Can you work these out from the model? Positions are in its coordinate system, mm. Face numbers are marked on the shaded views. A direction names the side the tool comes from. Give positions to 0.01 mm unless a question says otherwise; leave off trailing zeros. Write each loop counter-clockwise with the first axis right and the second up, starting at its lowest first coordinate (ties: lowest second). Pieces come first, ordered by that corner, then holes.
1. Suppose I cut it at A-A (z = 14.5). Please give me the cut outline in (x, y), and give its area (3 significant figures).
2. On a 3-axis mill with a long thin cutter (end or side, diameter ignored), from which of +Z, -Z, +X, -X, +Y, -Y can I reach the whole of each face in a straight line? I mean the marked faces 4, 5 and 6. Say none if no direction works.
3. I'm going to push flat-ended pins straight in: pin 1 (17.5 mm diameter, centred on x = 121.5, y = 19, fed in from +Z); pin 2 (6 mm diameter, centred on x = 19.5, y = 13.5, fed in from -Z); pin 3 (20.5 mm diameter, centred on x = 63.5, z = 59.69, fed in from -Y); pin 4 (8 mm diameter, centred on y = 51.5, z = 42.5, fed in from -X). Where does each tip first touch, or does it pass through?
4. Thinking about a two-plate mould opening in Z: for the marked faces 1, 2 and 3, which applies, pulls with the +Z half, pulls with the -Z half, needs draft (parallel to the pull), parting line crosses it, or undercut?
5. If I drill on probe 1 along Y at (x, z) = (63.5, 76.5) (3 decimals); probe 2 along X at (y, z) = (38, 9.5); probe 3 along Z at (x, y) = (21.5, 47.5), over which ranges is the centre line in solid material (lowest first)?
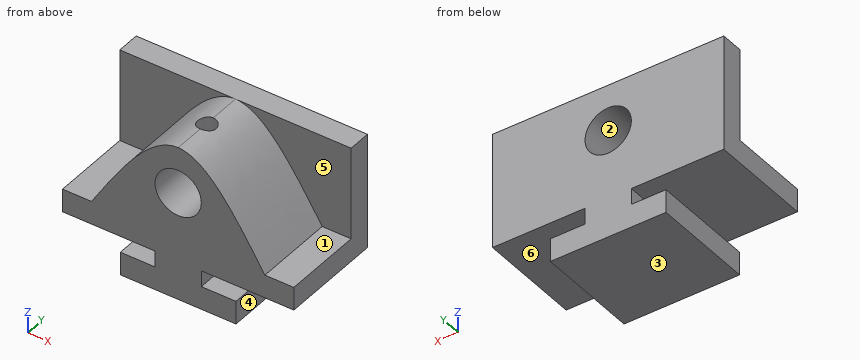
```python
from build123d import *

# Parameters (mm, degrees)
F0_W     = 127
F0_H     = 85.09
F1_DEPTH = 57.15
F2_R     = 12.7
F3_DEPTH = 57.15
F4_R     = 5.08
F5_DEPTH = 25.4
F6_DEPTH = 44.45


with BuildPart() as f1:
    # F0 (on Front) → F1 (new body)
    with BuildSketch(Plane.XZ):
        with Locations((63.5, 42.545)):
            Rectangle(F0_W, F0_H)
    extrude(amount=-F1_DEPTH)

    # F2 (on face) → F3 (cut)
    with BuildSketch(Plane.XZ):
        Polygon((95.25, 12.7), (95.25, 0), (127, 0), (127, 21.59), (76.2, 21.59), (76.2, 12.7), align=None)
        Polygon((0, 0), (31.75, 0), (31.75, 12.7), (50.8, 12.7), (50.8, 21.59), (0, 21.59), align=None)
        with Locations((63.5, 59.69)):
            Circle(F2_R)
    extrude(amount=-F3_DEPTH, mode=Mode.SUBTRACT)

    # F4 (on face) → F5 (cut)
    with BuildSketch(Plane.XY.offset(85.09)):
        with Locations((63.5, 22.225)):
            Circle(F4_R)
    extrude(amount=-F5_DEPTH, mode=Mode.SUBTRACT)

    # F2 (on face) → F6 (cut)
    with BuildSketch(Plane.XZ):
        with BuildLine():
            Line((0, 85.09), (0, 34.29))
            Line((0, 34.29), (15.875, 34.29))
            add(Edge.make_bspline(
                [(15.875, 34.29), (31.75, 59.69), (47.625, 85.09), (63.5, 85.09)],
                knots=[0, 0, 0, 0, 0.5, 0.5, 0.5, 0.5], degree=3))
            Line((63.5, 85.09), (0, 85.09))
        make_face()
        with BuildLine():
            Line((111.125, 34.29), (127, 34.29))
            Line((127, 34.29), (127, 85.09))
            Line((127, 85.09), (63.5, 85.09))
            add(Edge.make_bspline(
                [(63.5, 85.09), (79.375, 85.09), (95.25, 59.69), (111.125, 34.29)],
                knots=[0.5, 0.5, 0.5, 0.5, 1, 1, 1, 1], degree=3))
        make_face()
    extrude(amount=-F6_DEPTH, mode=Mode.SUBTRACT)


solid = f1.part
```
Checks:
1. outline: (50.8, 0) - (76.2, 0) - (76.2, 57.15) - (50.8, 57.15) - close
1. area: 1,450 mm2
2. face 4: -Z, +X, +Y, -Y
2. face 5: +Z, +X, -Y
2. face 6: +X, +Y, -Y
3. pin 1: stops at z = 34.29
3. pin 2: stops at z = 21.59
3. pin 3: passes through
3. pin 4: stops at x = 0
4. face 1: pulls with the +Z half
4. face 2: undercut
4. face 3: pulls with the -Z half
5. probe 1: y = 0 to 17.145, 27.305 to 57.15
5. probe 2: x = 31.75 to 95.25
5. probe 3: z = 21.59 to 85.09
